from build123d import *

# Parameters (mm, degrees)
F1_DEPTH    = 5
F2_R        = 1.75
F3_DEPTH    = 23.501
F4_T1_DEPTH = 15.1433659759
F4_T3_DEPTH = 16.1433659759
F4_T5_DEPTH = 13.1544598894
F5_R        = 2


# Not quite as in the source:
# - a fillet or chamfer that OpenCascade refuses, or shapes differently, is made with other operations: its cross-section is extruded or revolved along the edge and cut away or added


with BuildPart() as f1:
    # F0 (on Front) → F1 (new body, symmetric)
    with BuildSketch(Plane.XZ):
        Polygon((0, 3.5), (0, 0), (-11, 0), (-11, -20), (0, -20), (10, -1.5), (10, 3.5), align=None)
    extrude(amount=F1_DEPTH, both=True)

    # F2 (on face) → F3 (cut, through all)
    with BuildSketch(Plane.XY.offset(3.5)):
        with Locations((-6.5, 0)):
            Circle(F2_R)
        with Locations((5, 0)):
            Circle(F2_R)
    extrude(amount=-F3_DEPTH, mode=Mode.SUBTRACT)

    # F4: chamfer of 1 on 5 edges, made by hand

    # F4_s2 → F4_t1 (cut)
    with BuildSketch(Plane.XZ.offset(-7.571682988)):
        Polygon((-11, -19), (-10, -20), (-11, -20), align=None)
    extrude(amount=F4_T1_DEPTH, mode=Mode.SUBTRACT)

    # F4_s4 → F4_t3 (cut)
    with BuildSketch(Plane.YZ.offset(-13.571682988)):
        Polygon((5, -19), (4, -20), (5, -20), align=None)
        Polygon((-5, -19), (-4, -20), (-5, -20), align=None)
    extrude(amount=F4_T3_DEPTH, mode=Mode.SUBTRACT)

    # F4_s6 → F4_t5 (cut)
    with BuildSketch(Plane.XZ.offset(-6.5772299447)):
        Polygon((-0.5962022078, -20), (0.2835043057, -19.4755170344), (0, -20), align=None)
    extrude(amount=F4_T5_DEPTH, mode=Mode.SUBTRACT)

    # F4_s7 → F4_t8 (revolve, cut)
    with BuildSketch(Plane.XZ):
        Polygon((-3.75, -20), (-4.75, -19), (-4.75, -20), align=None)
    revolve(axis=Axis((-6.5, 0, -20), (0, 0, 1)), mode=Mode.SUBTRACT)

    # F5
    f5_edges = [f1.edges().sort_by_distance(p)[0] for p in [
        (-11, -5, -9.5),
        (-11, 5, -9.5),
        (5.27027, -5, -10.25),
        (10, -5, 1),
        (10, 5, 1),
        (5.27027, 5, -10.25),
    ]]
    fillet(f5_edges, radius=F5_R)


solid = f1.part
Verification items for the finished model (mm, model axes). A direction names the side the tool comes from. Round coordinates to 2 decimals unless told otherwise and drop trailing zeros. Loops run counter-clockwise (first coordinate to the right, second up) from the corner with the lowest first, then second, coordinate; pieces in that order, holes last. Notation, with made-up numbers: (63.5, 25) - (112.5, 25) arc R28 cw to (112.5, 53) - close; hole circle Ø3 at (-9.75, 78). An arc over 180 degrees is marked (long way). Use one line per item in the form item = value.
1. Section check C-C on y = 0. Record the cut outline in (x, z), and give its area (3 significant figures).
A:
outline = (-11, -19) - (-10, -20) - (-9.25, -20) - (-8.25, -19) - (-8.25, 0) - (-11, 0) - close; (-4.75, -19) - (-3.75, -20) - (-0.6, -20) - (0.28, -19.48) - (3.25, -13.99) - (3.25, 3.5) - (0, 3.5) - (0, 0) - (-4.75, 0) - close; (6.75, -7.51) - (10, -1.5) - (10, 3.5) - (6.75, 3.5) - close
area = 241 mm²
2. Draft check along Y on faces 3 (the flat face through (-10.5, 0.1, -19.5)), 4 (the flat face through (-5.4, -4.5, -19.5)), 5 (the cylindrical face through (-5.69, -1.55, -9.37)), 6 (the cylindrical face through (4.54, 4.43, -10.34)). Enter one of: pulls with the +Y half, pulls with the -Y half, needs draft (parallel to the pull), parting line crosses it, or undercut.
A:
face_3 = needs draft
face_4 = pulls with the -Y half
face_5 = undercut
face_6 = pulls with the +Y half
3. Section check B-B on z = 2.25. Record the cut outline in (x, y).
A:
outline = (0, -5) - (8, -5) arc R2 ccw to (10, -3) - (10, 3) arc R2 ccw to (8, 5) - (0, 5) - close; hole circle Ø3.5 at (5, 0)
4. Section check A-A on x = -6.5. Record the cut outline in (y, z).
A:
outline = (-5, -19) - (-4, -20) - (-2.75, -20) - (-1.75, -19) - (-1.75, 0) - (-5, 0) - close; (1.75, -19) - (2.75, -20) - (4, -20) - (5, -19) - (5, 0) - (1.75, 0) - close
5. Scan lines: probe 1 along Y at (x, z) = (-6.5, -13); probe 2 along X at (y, z) = (-1.25, -3.5); probe 3 along Z at (x, y) = (-6.25, 3.25). Record each from-to range of solid material in increasing order.
A:
probe_1 = -5 to -1.75, 1.75 to 5
probe_2 = -11 to -7.72, -5.28 to 3.78, 6.22 to 8.92
probe_3 = -20 to 0
6. Section check D-D on y = -3.5. Record the cut outline in (x, z), and give its area (3 significant figures).
A:
outline = (-10.94, -19.06) - (-10, -20) - (-0.6, -20) - (0.18, -19.54) - (9.94, -1.48) - (9.94, 3.5) - (0, 3.5) - (0, 0) - (-10.94, 0) - close
area = 359 mm²
7. Access from +Z, -Z, +X, -X, +Y, -Y to the whole of each face (thin tool, end or side, straight path). Record for faces 1 (the flat face through (0, 0, 2)), 2 (the cylindrical face through (4.54, -4.43, -10.34)).
A:
face_1 = +Z, -X, +Y, -Y
face_2 = -Z, +X, -Y
8. Gauge pin test, flat ends, axial feed: pin 1 Ø5 at (x, y) = (-3, 1.5) entering from +Z; pin 2 Ø3 at (x, y) = (-6.5, 0) entering from +Z; pin 3 Ø4 at (y, z) = (0, 2.5) entering from -X; pin 4 Ø2 at (y, z) = (0, -9.5) entering from +X. Record the tip position at first contact, or that the pin passes through.
A:
pin_1 = 0
pin_2 = through
pin_3 = 0
pin_4 = 3.56
